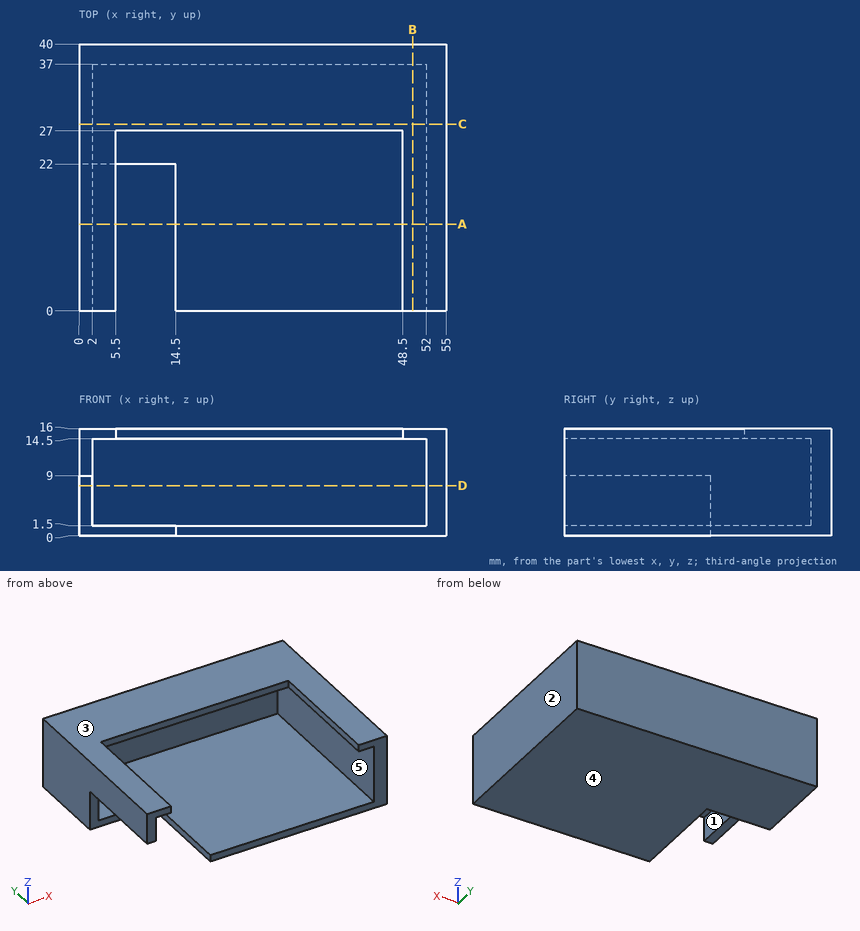
Part print with two shaded views. Sizes in mm from the minimum x, y, z corner. A direction names the side the tool comes from. Round coordinates to 2 decimals unless told otherwise and drop trailing zeros. Order: outer loops, then holes, each group sorted by start corner. A loop starts at its lowest first (then second) coordinate and runs counter-clockwise, first axis right, second up. Notation, with made-up numbers: M 73,7.25 L 117,7.25 A24 ccw 117,21.25 Z; hole C 47,-5 d4. An arc over 180 degrees is marked long. Answer in a Markdown table with one row per item. Add a question column.
Q1. Cut at A-A on y = 13. Give the cut face in (x, z).
Q2. Wall check: L1, parallel to Z at x = 43.5, y = 35.5; L2, parallel to X at y = 29, z = 9.25; L3, parallel to X at y = 14, z = 14.75. Give the ranges that are in metal, low to high. Write a range as from..to.
Q3. Cut at C-C on y = 28. Give the cut face in (x, z), and give its area (3 significant figures).
Q4. Pin check, flat tips, straight feed: pin 1 (1.6 mm diameter, centred on x = 35.5, z = 15, fed in from -Y); pin 2 (0.6 mm diameter, centred on x = 1, y = 14, fed in from -Z); pin 3 (3 mm diameter, centred on x = 39.5, z = 6, fed in from -Y). Stop position of each tip, or through.
Q5. Mould opens along X. For the marked faces 1, 2 and 3 say: +X half, -X half, draft (parallel to the pull), parting line (faces both ways), or undercut.
Q6. Cut at D-D on z = 7.5. Give the cut face in (x, y), and give its area (3 significant figures).
Q7. Cut at B-B on x = 50. Give the cut face in (y, z).
Q8. 3-axis set-ups, long thin cutter, end or side, ignore diameter. For the marked faces 4 and 5: which of +Z, -Z, +X, -X, +Y, -Y reach the whole face in a straight line?
Established:
| question | item | result |
|---|---|---|
| 1 | outline | M 0,9 L 2,9 L 2,14.5 L 5.5,14.5 L 5.5,16 L 0,16 Z; M 14.5,0 L 55,0 L 55,16 L 48.5,16 L 48.5,14.5 L 52,14.5 L 52,1.5 L 14.5,1.5 Z |
| 2 | L1 | z = 0..1.5, 14.5..16 |
| 2 | L2 | x = 0..2, 52..55 |
| 2 | L3 | x = 0..5.5, 48.5..55 |
| 3 | outline | M 0,0 L 55,0 L 55,16 L 0,16 Z; hole M 2,1.5 L 52,1.5 L 52,14.5 L 2,14.5 Z |
| 3 | area | 230 mm2 |
| 4 | pin 1 | stops at y = 27 |
| 4 | pin 2 | stops at z = 9 |
| 4 | pin 3 | stops at y = 37 |
| 5 | face 1 | undercut |
| 5 | face 2 | +X half |
| 5 | face 3 | draft |
| 6 | outline | M 0,22 L 2,22 L 2,37 L 52,37 L 52,0 L 55,0 L 55,40 L 0,40 Z |
| 6 | area | 306 mm2 |
| 7 | outline | M 0,0 L 40,0 L 40,16 L 0,16 L 0,14.5 L 37,14.5 L 37,1.5 L 0,1.5 Z |
| 8 | face 4 | -Z, +X, -X, +Y, -Y |
| 8 | face 5 | -Y |
